```python
from build123d import *

# Parameters (mm, degrees)
BOSS_EXTRUDE1_DEPTH = 10
SKETCH3_W           = 50
SKETCH3_H           = 2
SKETCH4_W           = 50
SKETCH4_H           = 2


with BuildPart() as part:
    # Sketch1 → Boss-Extrude1 (new body)
    with BuildSketch(Plane.XY):
        with BuildLine():
            Line((0, 0), (-120, 0))
            ThreePointArc((-120, 0), (-214.59995491, 16.200135269), (-300, 60))
            Line((-300, 60), (-300, 120))
            ThreePointArc((-300, 120), (-214.59995491, 163.799864731), (-120, 180))
            Line((-120, 180), (0, 180))
            ThreePointArc((0, 180), (-37.279220614, 90), (0, 0))
        make_face()
    extrude(amount=BOSS_EXTRUDE1_DEPTH)

    # Sweep2: sweep along a curve in space
    with BuildLine() as sweep2_path:
        ThreePointArc((0, 0, 0), (-37.279220614, 90, 0), (0, 180, 0))
    # 3DSketch2 → Sweep2 (sweep)
    with BuildSketch(Plane(origin=(0, 0, 0), x_dir=(-0.03996803834887158, 0, -0.9992009587217895), z_dir=(0, -1, 0))):
        Polygon((0, 0), (49.960047936, 1.998401917), (50.039984013, 0), (0.079936077, -1.998401917), align=None)
    sweep(path=sweep2_path.line)

    # Sweep3: sweep along a curve in space
    with BuildLine() as sweep3_path:
        ThreePointArc((-300, 60, 0), (-214.59995491, 16.200135269, 0), (-120, 0, 0))
    # Sketch3 → Sweep3 (sweep)
    with BuildSketch(Plane.ZY.offset(300)):
        with Locations((-25, 61)):
            Rectangle(SKETCH3_W, SKETCH3_H)
    sweep(path=sweep3_path.line)

    # Sweep4: sweep along a curve in space
    with BuildLine() as sweep4_path:
        ThreePointArc((-120, 180, 0), (-214.59995491, 163.799864731, 0), (-300, 120, 0))
    # Sketch4 → Sweep4 (sweep)
    with BuildSketch(Plane.ZY.offset(300)):
        with Locations((-25, 119)):
            Rectangle(SKETCH4_W, SKETCH4_H)
    sweep(path=sweep4_path.line)


solid = part.part
```
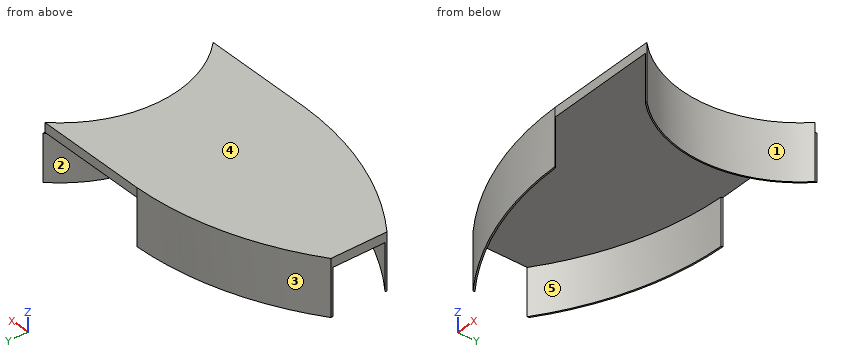
Geometry: final body of the model. Coordinates: model frame, mm. Face numbers are marked on the shaded views. A direction names the side the tool comes from. Coordinates: 2 decimals unless noted, no trailing zeros. Loops run counter-clockwise (first coordinate to the right, second up) from the corner with the lowest first, then second, coordinate; pieces in that order, holes last. Notation, with made-up numbers: (31.5, 60.25) -> (90.5, 60.25) arc R35 cw to (90.5, 98.25) -> close; hole circle Ø9 at (11.25, 79.25). An arc over 180 degrees is marked (long way). Use a Markdown table: item, result. Add a question column.
(1) Section query C-C, the plane y = 56. Return loops of the section in (x, z), plus the area to 3 significant figures.
(2) Section query A-A, the plane z = -30. Return loops of the section in (x, y).
(3) Line query: line 1 along Z through (x, y) = (-231, 125.5); line 2 along X through (y, z) = (91, -22.5); line 3 along Y through (x, z) = (-83.5, 5.5). Output: solid intervals per line, ascending.
(4) Mould query, pull axis Y, two halves, no side actions, for the marked faces 1, 2 and 3. Classes: pulls with the +Y half, pulls with the -Y half, needs draft (parallel to the pull), parting line crosses it, or undercut.
(5) Pin query (flat end, axial travel): pin 1 Ø1 at (y, z) = (135.5, -10) entering from +X; pin 2 Ø12 at (x, y) = (-259.5, 156.5) entering from -Z; pin 3 Ø11 at (x, z) = (-64.5, 4) entering from +Y; pin 4 Ø1 at (x, y) = (-137.5, 99.5) entering from -Z. Return the tip coordinate at first contact, or that it passes through.
(6) Section query B-B, the plane x = -180. Return loops of the section in (y, z), plus the area to 3 significant figures.
(7) Access query for the marked faces 4 and 5. Directions: +Z, -Z, +X, -X, +Y, -Y. A direction counts if a zero-diameter tool reaches every point of the face in a straight line with its end or side. Return the directions, or none.
(8) Section query D-D, the plane x = -93. Return loops of the section in (y, z), plus the area to 3 significant figures.
Answer:
| question | item | result |
|---|---|---|
| 1 | outline | (-294.34, -50) -> (-291.47, -50) -> (-291.47, 0) -> (-34.13, 0) -> (-34.13, -50) -> (-32.65, -50) -> (-32.65, 10) -> (-294.34, 10) -> close |
| 1 | area | 2,830 mm^2 |
| 2 | outline | (-300, 60) arc R316.63 ccw to (-120, 0) -> (-121.14, 1.64) arc R315.01 cw to (-300, 62) -> close; (-300, 118) arc R315.01 cw to (-121.14, 178.36) -> (-120, 180) arc R316.63 ccw to (-300, 120) -> close; (-2, 0) -> (0, 0) arc R127.28 cw to (0, 180) -> (0, 182) arc R128.7 ccw to start |
| 3 | line 1 | z = 0 to 10 |
| 3 | line 2 | x = -38.7 to -37.28 |
| 3 | line 3 | y = 0 to 180 |
| 4 | face 1 | undercut |
| 4 | face 2 | parting line crosses it |
| 4 | face 3 | pulls with the +Y half |
| 5 | pin 1 | stops at x = -28.68 |
| 5 | pin 2 | passes through |
| 5 | pin 3 | stops at y = 180 |
| 5 | pin 4 | stops at z = 0 |
| 6 | outline | (6.81, -50) -> (8.46, -50) -> (8.46, 0) -> (171.54, 0) -> (171.54, -50) -> (173.19, -50) -> (173.19, 10) -> (6.81, 10) -> close |
| 6 | area | 1,830 mm^2 |
| 7 | face 4 | +Z, +X, -X, +Y, -Y |
| 7 | face 5 | -Z |
| 8 | outline | (0, 0) -> (180, 0) -> (180, 10) -> (0, 10) -> close |
| 8 | area | 1,800 mm^2 |
